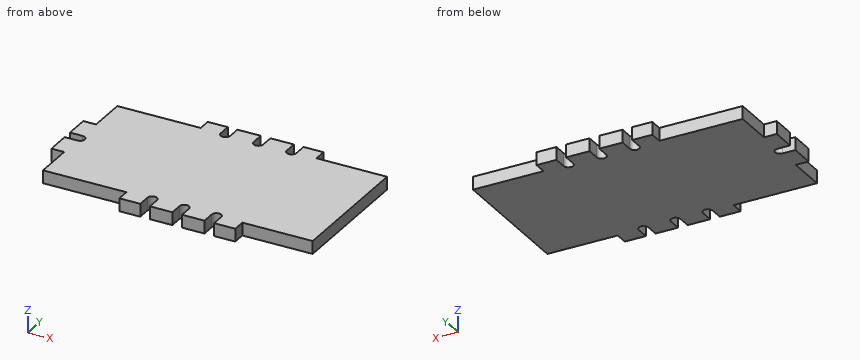
```python
from build123d import *

# Parameters (mm, degrees)
F0_W      = 279.4
F0_H      = 158.75
F1_DEPTH  = 12.7
F2_W      = 12.7
F2_H      = 50.8
F3_DEPTH  = 12.701
F5_DEPTH  = 12.701
F6_W      = 69.85
F6_H      = 12.7
F6_W_2    = 82.55
F7_DEPTH  = 12.701
F9_DEPTH  = 12.701
F10_DEPTH = 12.701


with BuildPart() as f1:
    # F0 (on Top) → F1 (new body)
    with BuildSketch(Plane.XY):
        with Locations((139.7, 79.375)):
            Rectangle(F0_W, F0_H)
    extrude(amount=-F1_DEPTH)

    # F2 (on Top) → F3 (cut, through all)
    with BuildSketch(Plane.XY):
        with Locations((6.35, 133.423964)):
            Rectangle(F2_W, F2_H)
        with Locations((6.35, 25.4)):
            Rectangle(F2_W, F2_H)
    extrude(amount=-F3_DEPTH, mode=Mode.SUBTRACT)

    # F4 (on Top) → F5 (cut, through all)
    with BuildSketch(Plane.XY):
        with BuildLine():
            Line((0, 74.611429), (12.700348, 74.6125))
            ThreePointArc((12.700348, 74.6125), (17.462176, 79.425701), (12.598951, 84.136429))
            Line((12.598951, 84.136429), (0, 84.136429))
            Line((0, 84.136429), (0, 74.611429))
        make_face()
    extrude(amount=-F5_DEPTH, mode=Mode.SUBTRACT)

    # F6 (on Top) → F7 (cut, through all)
    with BuildSketch(Plane.XY):
        with Locations((244.747044, 6.35)):
            Rectangle(F6_W, F6_H)
        with Locations((53.942362, 6.35)):
            Rectangle(F6_W_2, F6_H)
        with Locations((53.887489, 152.495061)):
            Rectangle(F6_W_2, F6_H)
        with Locations((244.602786, 152.552579)):
            Rectangle(F6_W, F6_H)
    extrude(amount=-F7_DEPTH, mode=Mode.SUBTRACT)

    # F8 (on Top) → F9 (cut, through all)
    with BuildSketch(Plane.XY):
        with BuildLine():
            Line((147.625268, 158.788487), (147.637502, 146.045427))
            ThreePointArc((147.637502, 146.045427), (152.40284, 141.287501), (157.1625, 146.051108))
            Line((157.1625, 146.051108), (157.1625, 158.788487))
            Line((157.1625, 158.788487), (147.625268, 158.788487))
        make_face()
        with BuildLine():
            Line((157.159752, 0), (157.159752, 12.538237))
            ThreePointArc((157.159752, 12.538237), (152.493737, 17.461577), (147.637569, 12.725692))
            ThreePointArc((147.637569, 12.725692), (147.6375, 12.7), (147.637569, 12.674308))
            Line((147.637569, 12.674308), (147.637569, 0))
            Line((147.637569, 0), (157.159752, 0))
        make_face()
    extrude(amount=-F9_DEPTH, mode=Mode.SUBTRACT)

    # F8 (on Top) → F10 (cut, through all)
    with BuildSketch(Plane.XY):
        with BuildLine():
            Line((157.159752, 0), (157.159752, 12.538237))
            ThreePointArc((157.159752, 12.538237), (152.493737, 17.461577), (147.637569, 12.725692))
            ThreePointArc((147.637569, 12.725692), (147.6375, 12.7), (147.637569, 12.674308))
            Line((147.637569, 12.674308), (147.637569, 0))
            Line((147.637569, 0), (157.159752, 0))
        make_face()
        with BuildLine():
            Line((188.9125, 0), (188.9125, 12.7))
            ThreePointArc((188.9125, 12.7), (184.15, 17.4625), (179.3875, 12.7))
            Line((179.3875, 12.7), (179.3875, 0))
            Line((179.3875, 0), (188.9125, 0))
        make_face()
        with BuildLine():
            Line((125.4125, 0), (125.4125, 12.7))
            ThreePointArc((125.4125, 12.7), (120.65, 17.4625), (115.8875, 12.7))
            Line((115.8875, 12.7), (115.8875, 0))
            Line((115.8875, 0), (125.4125, 0))
        make_face()
        with BuildLine():
            Line((115.036184, 158.751108), (115.03323, 146.051108))
            ThreePointArc((115.03323, 146.051108), (119.795176, 141.2875), (124.55823, 146.05))
            Line((124.55823, 146.05), (124.55823, 158.751108))
            Line((124.55823, 158.751108), (115.036184, 158.751108))
        make_face()
        with BuildLine():
            Line((147.625268, 158.788487), (147.637502, 146.045427))
            ThreePointArc((147.637502, 146.045427), (152.40284, 141.287501), (157.1625, 146.051108))
            Line((157.1625, 146.051108), (157.1625, 158.788487))
            Line((157.1625, 158.788487), (147.625268, 158.788487))
        make_face()
        with BuildLine():
            Line((180.360956, 158.751108), (180.363911, 146.05))
            ThreePointArc((180.363911, 146.05), (185.126964, 141.2875), (189.88891, 146.051108))
            Line((189.88891, 146.051108), (189.885956, 158.751108))
            Line((189.885956, 158.751108), (180.360956, 158.751108))
        make_face()
    extrude(amount=-F10_DEPTH, mode=Mode.SUBTRACT)


solid = f1.part
```
Geometry check sheet. Reference: the model listing, model coordinates, mm. Round coordinates to 2 decimals unless told otherwise and drop trailing zeros. Order: outer loops, then holes, each group sorted by start corner. A loop starts at its lowest first (then second) coordinate and runs counter-clockwise, first axis right, second up. Notation, with made-up numbers: M 41.25,-13 L 64.25,-13 A28 cw 64.25,14 Z; hole C -34,47.5 d7. An arc over 180 degrees is marked long. Answer as CSV lines item,"result".
1) Gauge pin test, flat ends, axial feed: pin 1 Ø6.5 at (y, z) = (155.5, -9) entering from +X; pin 2 Ø6.5 at (y, z) = (8, -4.5) entering from +X; pin 3 Ø5 at (y, z) = (127.5, -6) entering from -X. Record the tip position at first contact, or that the pin passes through.
Entries:
pin 1,"x = 209.68"
pin 2,"x = 209.82"
pin 3,"x = 12.7"
2) Sectioned sample at B-B on y = 111. Record the cut outline in (x, z), and give its area (3 significant figures).
Entries:
outline,"M 12.7,-12.7 L 279.4,-12.7 L 279.4,0 L 12.7,0 Z"
area,"3,390 mm2"
3) Sectioned sample at A-A on x = 225.5. Record the cut outline in (y, z), and give its area (3 significant figures).
Entries:
outline,"M 12.7,-12.7 L 146.2,-12.7 L 146.2,0 L 12.7,0 Z"
area,"1,700 mm2"
4) Thickness scan on probe 1 along X at (y, z) = (8.5, -6); probe 2 along Y at (x, z) = (244.5, -10.5); probe 3 along X at (y, z) = (121, -1.75). Record the ranges inside material, lowest first. Write a range as [from, to].
Entries:
probe 1,"[95.22, 115.89], [125.41, 147.64], [157.16, 179.39], [188.91, 209.82]"
probe 2,"[12.7, 146.2]"
probe 3,"[12.7, 279.4]"
